Part print with two shaded views. Sizes in mm from the minimum x, y, z corner. A direction names the side the tool comes from. Round coordinates to 2 decimals unless told otherwise and drop trailing zeros. Order: outer loops, then holes, each group sorted by start corner. A loop starts at its lowest first (then second) coordinate and runs counter-clockwise, first axis right, second up. Notation, with made-up numbers: M -5,87.5 L 0,87.5 A8 cw 0,100.5 Z; hole C 40,49 d7. An arc over 180 degrees is marked long. Answer as a JSON object with one key per item and string values.
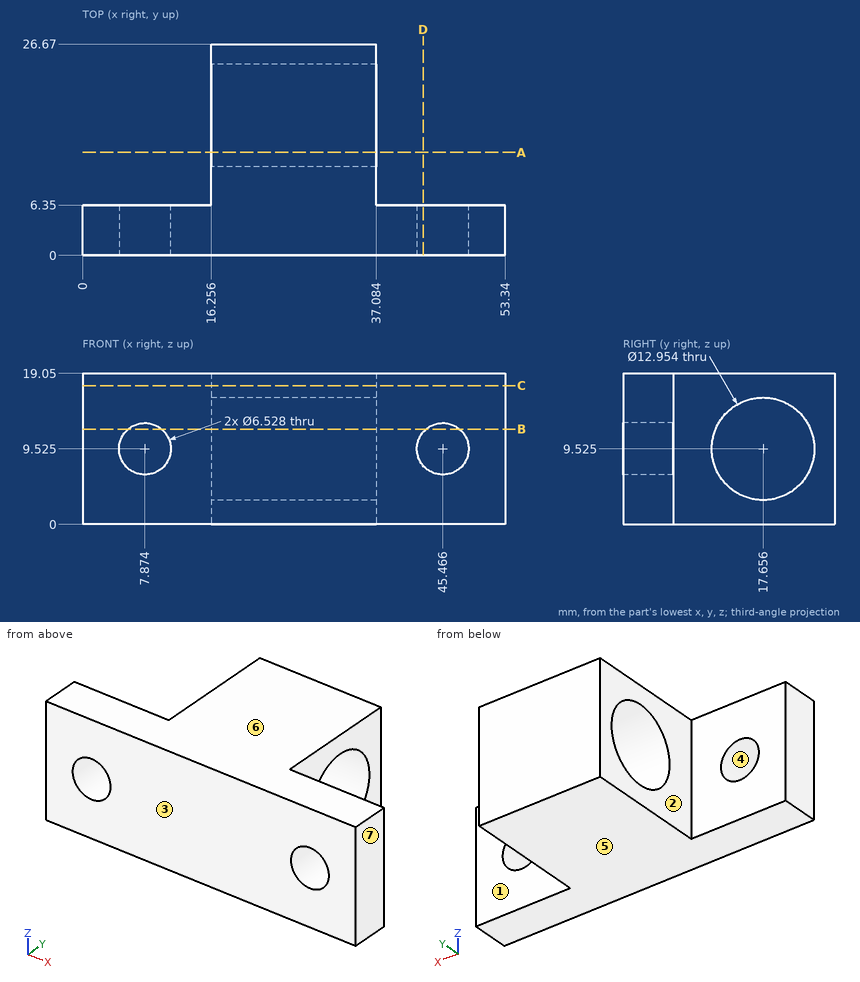
Item 1: Saw through at C-C on z = 17.5. List the corners of the cut face in (x, y).
Worked answers:
{"outline": "M 0,0 L 53.34,0 L 53.34,6.35 L 37.08,6.35 L 37.08,26.67 L 16.26,26.67 L 16.26,6.35 L 0,6.35 Z"}
Item 2: Saw through at D-D on x = 43. List the corners of the cut face in (y, z).
Worked answers:
{"outline": "M 0,0 L 6.35,0 L 6.35,7.39 L 0,7.39 Z; M 0,11.66 L 6.35,11.66 L 6.35,19.05 L 0,19.05 Z"}
Item 3: Saw through at A-A on y = 13. List the corners of the cut face in (x, z).
Worked answers:
{"outline": "M 16.26,0 L 37.08,0 L 37.08,5.02 L 16.26,5.02 Z; M 16.26,14.03 L 37.08,14.03 L 37.08,19.05 L 16.26,19.05 Z"}
Item 4: Wall check: line 1 along X through (y, z) = (5, 8.25); line 2 along X through (y, z) = (11.75, 12.5); line 3 along Y through (x, z) = (27, 7.75) (1 decimal). Give the ranges that are in metal, low to high. Write a range as [from, to].
Worked answers:
{"line 1": "x = [0, 4.87], [10.88, 42.46], [48.47, 53.34]", "line 2": "x = [16.26, 37.08]", "line 3": "y = [0, 11.4], [23.9, 26.7]"}
Item 5: Drop flat-ended pins along their axis: pin 1 Ø5 at (y, z) = (15.5, 15.5) entering from -X; pin 2 Ø5 at (x, z) = (44.5, 6) entering from +Y. Give the stop position or say it passes through.
Worked answers:
{"pin 1": "stops at x = 16.26", "pin 2": "stops at y = 6.35"}
Item 6: Saw through at B-B on z = 12. List the corners of the cut face in (x, y).
Worked answers:
{"outline": "M 0,0 L 5.75,0 L 5.75,6.35 L 0,6.35 Z; M 10,0 L 43.34,0 L 43.34,6.35 L 37.08,6.35 L 37.08,11.67 L 16.26,11.67 L 16.26,6.35 L 10,6.35 Z; M 16.26,23.64 L 37.08,23.64 L 37.08,26.67 L 16.26,26.67 Z; M 47.59,0 L 53.34,0 L 53.34,6.35 L 47.59,6.35 Z"}
Item 7: 3-axis set-ups, long thin cutter, end or side, ignore diameter. For the marked faces 1, 2 and 3: which of +Z, -Z, +X, -X, +Y, -Y reach the whole face in a straight line?
Worked answers:
{"face 1": "+Z, -Z, +X, +Y", "face 2": "+Z, -Z, -X, +Y", "face 3": "+Z, -Z, +X, -X, -Y"}
Item 8: Two-plate mould, pull along Z, no slides. Class the marked faces 4, 5, 6 and 7: released by +Z, released by -Z, zero draft, split by the parting line, or undercut.
Worked answers:
{"face 4": "undercut", "face 5": "released by -Z", "face 6": "released by +Z", "face 7": "zero draft"}
